Geometry: see drawing. Coordinates: mm, zero at the bounding-box minimum. A direction names the side the tool comes from. Coordinates: 2 decimals unless noted, no trailing zeros. Order: outer loops, then holes, each group sorted by start corner. A loop starts at its lowest first (then second) coordinate and runs counter-clockwise, first axis right, second up. Notation, with made-up numbers: (-7, 34) -> (21, 34) arc R11 cw to (21, 41) -> close; hole circle Ø11 at (80.25, -28). An arc over 180 degrees is marked (long way). Use one line per item in the form item = value.
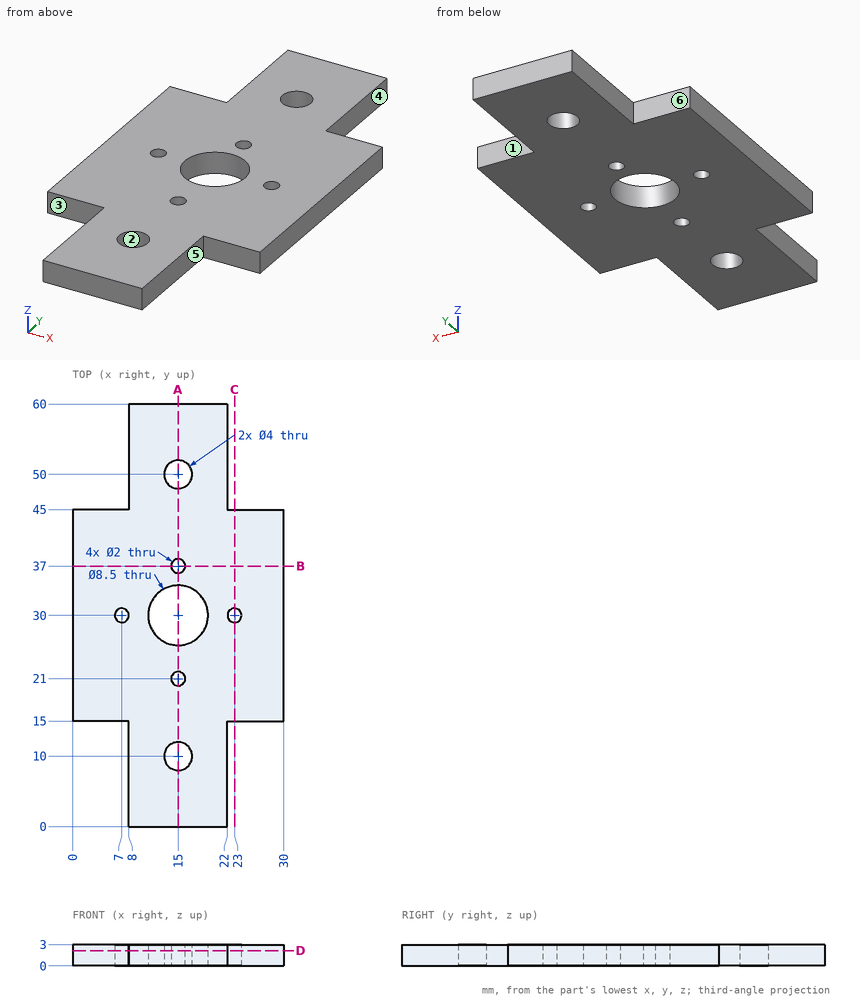
1) Contact query for flat-ended pins moving along their axis: P1, Ø1.5, axis at y = 11, z = 2, coming from the -X side; P2, Ø5, axis at x = 15, y = 30, coming from the +Z side; P3, Ø0.9, axis at x = 4, z = 2, coming from the +Y side; P4, Ø1.5, axis at y = 52, z = 2, coming from the +X side. Output: stop coordinate, or through.
Results found:
P1 = 8
P2 = through
P3 = 45
P4 = 22
2) Section D-D, the plane z = 2.15. Output: boundary loops of the cut face in (x, y).
Results found:
outline = (0, 15) -> (8, 15) -> (8, 0) -> (22, 0) -> (22, 15) -> (30, 15) -> (30, 45) -> (22, 45) -> (22, 60) -> (8, 60) -> (8, 45) -> (0, 45) -> close; hole circle Ø2 at (7, 30); hole circle Ø8.5 at (15, 30); hole circle Ø4 at (15, 10); hole circle Ø4 at (15, 50); hole circle Ø2 at (15, 21); hole circle Ø2 at (15, 37); hole circle Ø2 at (23, 30)
3) Section B-B, the plane y = 37. Output: boundary loops of the cut face in (x, z).
Results found:
outline = (0, 0) -> (14, 0) -> (14, 3) -> (0, 3) -> close; (16, 0) -> (30, 0) -> (30, 3) -> (16, 3) -> close
4) Access query for the marked faces 4, 5 and 6. Directions: +Z, -Z, +X, -X, +Y, -Y. A direction counts if a zero-diameter tool reaches every point of the face in a straight line with its end or side. Return the directions, or none.
Results found:
face_4 = +Z, -Z, +X, +Y
face_5 = +Z, -Z, +X, -Y
face_6 = +Z, -Z, -X, +Y
5) Pull-direction query (Y, two-part tool) for the marked faces 1, 2 and 3; classes: released by +Y, released by -Y, zero draft, split by the parting line, or undercut.
Results found:
face_1 = released by +Y
face_2 = undercut
face_3 = released by -Y
6) Section C-C, the plane x = 23. Output: boundary loops of the cut face in (y, z).
Results found:
outline = (15, 0) -> (29, 0) -> (29, 3) -> (15, 3) -> close; (31, 0) -> (45, 0) -> (45, 3) -> (31, 3) -> close
7) Material intervals for probe 1 along Y at (x, z) = (15, 2); probe 2 along Y at (x, z) = (7, 0.85); probe 3 along X at (y, z) = (53, 0.75), sorted ascending. Write a range as from..to.
Results found:
probe_1 = 0..8, 12..20, 22..25.75, 34.25..36, 38..48, 52..60
probe_2 = 15..29, 31..45
probe_3 = 8..22
8) Section A-A, the plane x = 15. Output: boundary loops of the cut face in (y, z), and give its area (4 significant figures).
Results found:
outline = (0, 0) -> (8, 0) -> (8, 3) -> (0, 3) -> close; (12, 0) -> (20, 0) -> (20, 3) -> (12, 3) -> close; (22, 0) -> (25.75, 0) -> (25.75, 3) -> (22, 3) -> close; (34.25, 0) -> (36, 0) -> (36, 3) -> (34.25, 3) -> close; (38, 0) -> (48, 0) -> (48, 3) -> (38, 3) -> close; (52, 0) -> (60, 0) -> (60, 3) -> (52, 3) -> close
area = 118.5 mm2
